For this review, take the finished solid that the model builds, in its own axes (mm). Face numbers are marked on the shaded views. A direction names the side the tool comes from. Coordinates: 2 decimals unless noted, no trailing zeros. Loops run counter-clockwise (first coordinate to the right, second up) from the corner with the lowest first, then second, coordinate; pieces in that order, holes last. Notation, with made-up numbers: (75, 20.25) -> (107, 20.25) arc R14 ccw to (107, 35.25) -> close; hole circle Ø2 at (15.25, 4.25). An arc over 180 degrees is marked (long way). Use a Markdown table: item, result.
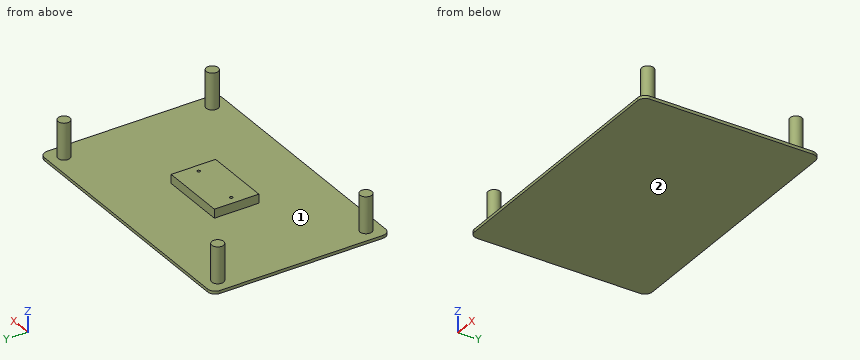
Autodesk Fusion 360 part; units mm, degrees
sketch "Sketch1" plane through (0, 0, 0) normal (0, 0, 1) x (1, 0, 0)
  line L0 (90, -60) -> (-90, -60)
  line L1 (-90, -60) -> (-90, 60)
  line L2 (-90, 60) -> (90, 60)
  line L3 (90, 60) -> (90, -60)
  line L4 (90, -60) -> (-90, 60) construction
  line L5 (-90, -60) -> (90, 60) construction
  circle A0 centre (-80, 50) radius 5
  circle A1 centre (-80, -50) radius 5
  circle A2 centre (80, 50) radius 5
  circle A3 centre (80, -50) radius 5
  dimension "d1" = 180
  dimension "d2" = 120
  dimension "d3" = 10
  dimension "d4" = 10
  dimension "d5" = 10
  dimension "d6" = 10
sketch "Sketch2" plane through (0, 0, 0) normal (0, 0, 1) x (1, 0, 0)
  line L0 (90, -60) -> (-90, -60)
  line L1 (-90, -60) -> (-90, 60)
  line L2 (-90, 60) -> (90, 60)
  line L3 (90, 60) -> (90, -60)
  line L4 (90, -60) -> (-90, 60) construction
  line L5 (-90, -60) -> (90, 60) construction
  dimension "d9" = 180
  dimension "d10" = 120
extrude "Extrude2" add sketch "Sketch2" along normal blind 5 makes body 1
sketch "Sketch3" plane through (0, 0, 5) normal (0, 0, 1) x (-1, 0, 0)
  line L0 (-90, -60) -> (90, -60)
  line L1 (90, -60) -> (90, 60)
  line L2 (90, 60) -> (-90, 60)
  line L3 (-90, 60) -> (-90, -60)
sketch "Sketch4" plane through (0, 0, 5) normal (0, 0, 1) x (-1, 0, 0)
  circle A0 centre (-80, 50) radius 4
  circle A1 centre (80, 50) radius 4
  circle A2 centre (-80, -50) radius 4
  circle A3 centre (80, -50) radius 4
  dimension "d13" = 8
  dimension "d14" = 8
  dimension "d15" = 8
  dimension "d16" = 8
extrude "Extrude3" add sketch "Sketch4" along normal blind 50 bodies 1
sketch "Sketch5" plane through (0, 0, 5) normal (0, 0, 1) x (-1, 0, 0)
  line L0 (22.5, -15) -> (-22.5, -15)
  line L1 (-22.5, -15) -> (-22.5, 15)
  line L2 (-22.5, 15) -> (22.5, 15)
  line L3 (22.5, 15) -> (22.5, -15)
  line L4 (22.5, -15) -> (-22.5, 15) construction
  line L5 (-22.5, -15) -> (22.5, 15) construction
  dimension "d19" = 45
  dimension "d20" = 30
extrude "Extrude4" add sketch "Sketch5" along normal blind 10 bodies 1
sketch "Sketch6" plane through (0, 0, 15) normal (0, 0, 1) x (-1, 0, 0)
  line L0 (22.5, 15) -> (-22.5, 15)
  line L1 (-22.5, 15) -> (-22.5, -15)
  line L2 (-22.5, -15) -> (22.5, -15)
  line L3 (22.5, -15) -> (22.5, 15)
  circle A0 centre (17, 0) radius 1
  circle A1 centre (-17, 0) radius 1
  dimension "d23" = 17
  dimension "d24" = 17
  dimension "d25" = 2
  dimension "d26" = 2
extrude "Extrude5" cut sketch "Sketch6" against normal blind 9 contours A0 | A1 bodies 1
extrude "Extrude6" cut 4 faces at (77.7042, -51.1056, 55) (77.7042, 48.8944, 55) (-82.2958, 48.8944, 55) (-82.2958, -51.1056, 55) along direction (0, 0, -1) blind 10 on bodies 1 bodies 1
extrude "Extrude7" cut 1 faces at (-5.4223, 10.2267, 15) along direction (0, 0, -1) blind 10 on bodies 1 bodies 1
extrude "Extrude8" cut sketch "Sketch3" against normal blind 3 bodies 1 makes body 2 at (-17.995, 0.0996, 5.3333) makes body 3 at (16.005, 0.0996, 5.3333) makes body 4 at (76.0199, -49.6017, 18.3333) makes body 5 at (-83.9801, -49.6017, 18.3333) makes body 6 at (76.0199, 50.3983, 18.3333) makes body 7 at (30, -20, 0)
extrude "Extrude9" add 1 faces at (-82.2958, 48.8944, 5) along direction (0, 0, -1) blind 3 on bodies 1 bodies 1 7
extrude "Extrude10" add 3 faces at (-82.2958, -51.1056, 5) (77.7042, -51.1056, 5) (77.7042, 48.8944, 5) along direction (0, 0, -1) blind 3 on bodies 4 5 6 bodies 5 1 4 6
sketch "Sketch7" plane through (0, 0, 2) normal (0, 0, 1) x (-1, 0, 0)
  circle A0 centre (-80, -50) radius 4
  circle A1 centre (80, 50) radius 4
  circle A2 centre (-80, 50) radius 4
  circle A3 centre (80, -50) radius 4
  line L0 (-90, 60) -> (-90, -60)
  line L1 (-90, -60) -> (90, -60)
  line L2 (90, -60) -> (90, 60)
  line L3 (90, 60) -> (-90, 60)
  line L4 (22.5, 15) -> (-22.5, 15)
  line L5 (-22.5, 15) -> (-22.5, -15)
  line L6 (-22.5, -15) -> (22.5, -15)
  line L7 (22.5, -15) -> (22.5, 15)
  line L8 (22.5, 15) -> (-22.5, -15) construction
  line L9 (-22.5, 15) -> (22.5, -15) construction
  dimension "d39" = 45
  dimension "d40" = 30
extrude "Extrude11" add sketch "Sketch7" along normal blind 6 contours L4 L5 L6 L7 bodies 2 3 5
sketch "Sketch8" plane through (0, 0, 8) normal (0, 0, 1) x (-1, 0, 0)
  line L0 (22.5, -15) -> (22.5, 15)
  line L1 (22.5, 15) -> (-22.5, 15)
  line L2 (-22.5, 15) -> (-22.5, -15)
  line L3 (-22.5, -15) -> (22.5, -15)
  circle A0 centre (-17, 0) radius 1
  circle A1 centre (17, 0) radius 1
  dimension "d43" = 17
  dimension "d44" = 17
  dimension "d45" = 2
  dimension "d46" = 2
extrude "Extrude12" cut sketch "Sketch8" against normal blind 7 contours A0 | A1 bodies 2
extrude "Extrude13" cut 4 faces at (77.7042, 48.8944, 45) (77.7042, -51.1056, 45) (-82.2958, -51.1056, 45) (-82.2958, 48.8944, 45) along direction (0, 0, -1) blind 10 on bodies 2 bodies 2
extrude "Extrude14" cut 4 faces at (77.7042, -51.1056, 35) (77.7042, 48.8944, 35) (-82.2958, 48.8944, 35) (-82.2958, -51.1056, 35) along direction (0, 0, -1) blind 8.5 on bodies 2 bodies 2
fillet "Fillet1" radius 5 4 edges at (-90, 60, 1) (-90, -60, 1) (90, -60, 1) (90, 60, 1) on bodies 1 2 5 7
sketch "Sketch9" plane through (0, 0, 2) normal (0, 0, 1) x (-1, 0, 0)
  circle A0 centre (80, 150) radius 5
  circle A1 centre (-80, 150) radius 5
  circle A2 centre (80, 250) radius 5
  circle A3 centre (-80, 250) radius 5
  line L0 (-90, 140) -> (90, 140)
  line L1 (90, 140) -> (90, 260)
  line L2 (90, 260) -> (-90, 260)
  line L3 (-90, 260) -> (-90, 140)
sketch "Sketch10" plane through (0, 0, 2) normal (0, 0, 1) x (-1, 0, 0)
  circle A0 centre (80, 150) radius 4.5
  circle A1 centre (-80, 150) radius 4.5
  circle A2 centre (80, 250) radius 4.5
  circle A3 centre (-80, 250) radius 4.5
  circle A4 centre (80, 250) radius 5.5
  circle A5 centre (80, 150) radius 5.5
  circle A6 centre (-80, 150) radius 5.5
  circle A7 centre (-80, 250) radius 5.5
  circle A8 centre (-80, 150) radius 5
  circle A9 centre (80, 250) radius 5
  circle A10 centre (80, 150) radius 5
  circle A11 centre (-80, 250) radius 5
  dimension "d59" = 9
  dimension "d60" = 9
  dimension "d61" = 9
  dimension "d62" = 9
  dimension "d63" = 11
  dimension "d64" = 11
  dimension "d65" = 11
  dimension "d66" = 11
(1) Take a section at A-A on x = 80. Write out the cut boundary in (y, z), plus the area to 3 significant figures.
Found:
| item | result |
|---|---|
| outline | (-60, 0) -> (60, 0) -> (60, 2) -> (54, 2) -> (54, 26.5) -> (46, 26.5) -> (46, 2) -> (-46, 2) -> (-46, 26.5) -> (-54, 26.5) -> (-54, 2) -> (-60, 2) -> close |
| area | 632 mm^2 |
(2) For pin 1 Ø1.8 at (y, z) = (-1, 5.5) entering from -X; pin 2 Ø1.8 at (x, z) = (-1, 5) entering from +Y; pin 3 Ø6.5 at (x, z) = (5, 6) entering from -Y, all flat-tipped, find the tip position at first contact; note any pin that passes through.
Found:
| item | result |
|---|---|
| pin 1 | stops at x = -22.5 |
| pin 2 | stops at y = 15 |
| pin 3 | stops at y = -15 |
(3) For line 1 along X through (y, z) = (0, 6); line 2 along Y through (x, z) = (17, 5.25); line 3 along Z through (x, y) = (57, -38), list the stretches that pass through material, from the lowest coordinate up.
Found:
| item | result |
|---|---|
| line 1 | x = -22.5 to -18, -16 to 16, 18 to 22.5 |
| line 2 | y = -15 to -1, 1 to 15 |
| line 3 | z = 0 to 2 |
(4) Take a section at B-B on y = 50. Write out the cut boundary in (x, z).
Found:
| item | result |
|---|---|
| outline | (-90, 0) -> (90, 0) -> (90, 2) -> (84, 2) -> (84, 26.5) -> (76, 26.5) -> (76, 2) -> (-76, 2) -> (-76, 26.5) -> (-84, 26.5) -> (-84, 2) -> (-90, 2) -> close |
(5) Take a section at D-D on x = 10.5. Write out the cut boundary in (y, z).
Found:
| item | result |
|---|---|
| outline | (-60, 0) -> (60, 0) -> (60, 2) -> (15, 2) -> (15, 8) -> (-15, 8) -> (-15, 2) -> (-60, 2) -> close |
(6) For the marked faces 1 and 2, list the 3-axis set-ups (+Z, -Z, +X, -X, +Y, -Y) from which the entire face can be reached by the end or side of a thin tool; tool diameter is ignored.
Found:
| item | result |
|---|---|
| face 1 | +Z |
| face 2 | -Z, +X, -X, +Y, -Y |
(7) Take a section at C-C on z = 20.25. Write out the cut boundary in (x, y).
Found:
| item | result |
|---|---|
| outline | circle Ø8 at (-80, -50); circle Ø8 at (-80, 50); circle Ø8 at (80, -50); circle Ø8 at (80, 50) |
